from build123d import *

# Parameters (mm, degrees)
F1_DEPTH       = 10
F3_DEPTH       = 10.001
F5_D           = 8.5
F5_CBORE_D     = 11
F5_CBORE_DEPTH = 2
F4_R           = 1.895
F6_DEPTH       = 1.5
F7_R           = 2
F9_DEPTH       = 4


with BuildPart() as f1:
    # F0 (on Front) → F1 (new body, symmetric)
    with BuildSketch(Plane.XZ):
        with BuildLine():
            Line((30, 51.9615242271), (0, 0))
            Line((0, 0), (130, 0))
            Line((130, 0), (130, 10))
            Line((130, 10), (88.031548244, 10))
            ThreePointArc((88.031548244, 10), (82.855167342, 10.6814834742), (78.031548244, 12.6794919243))
            Line((78.031548244, 12.6794919243), (60.9383223748, 22.5482704812))
            Line((60.9383223748, 22.5482704812), (62.1883223748, 24.7133339907))
            Line((62.1883223748, 24.7133339907), (44.8678142991, 34.7133339907))
            Line((44.8678142991, 34.7133339907), (43.6178142991, 32.5482704812))
            Line((43.6178142991, 32.5482704812), (26.2973062234, 42.5482704812))
            Line((26.2973062234, 42.5482704812), (31.2990381057, 51.2115242271))
            Line((31.2990381057, 51.2115242271), (30, 51.9615242271))
        make_face()
        with BuildLine():
            ThreePointArc((78.2347422219, 10.8301270189), (80.5643713533, 5.2059047745), (75.7347422219, 1.5))
            Line((75.7347422219, 1.5), (27.3774332424, 1.5))
            Line((27.3774332424, 1.5), (13.1251234055, 9.7387149337))
            ThreePointArc((13.1251234055, 9.7387149337), (10.7974587698, 12.7747007163), (11.2973058678, 16.5675077516))
            Line((11.2973058678, 16.5675077516), (23.0473062234, 36.9191053566))
            ThreePointArc((23.0473062234, 36.9191053566), (26.0833380169, 39.2487344881), (29.8774332424, 38.7492323755))
            Line((29.8774332424, 38.7492323755), (78.2347422219, 10.8301270189))
        make_face(mode=Mode.SUBTRACT)
    extrude(amount=F1_DEPTH, both=True)

    # F2 (on face) → F3 (cut, through all)
    with BuildSketch(Plane.XY.offset(10)):
        with BuildLine():
            Line((130, -10), (130, -5))
            Line((130, -5), (95, -5))
            ThreePointArc((95, -5), (92.2613872125, -6.7752551286), (92.7639320225, -10))
            Line((92.7639320225, -10), (130, -10))
        make_face()
        with BuildLine():
            ThreePointArc((92.7639320225, 10), (92.2613872125, 6.7752551286), (95, 5))
            Line((95, 5), (130, 5))
            Line((130, 5), (130, 10))
            Line((130, 10), (92.7639320225, 10))
        make_face()
        with BuildLine():
            Line((130, -3), (130, 3))
            Line((130, 3), (113, 3))
            ThreePointArc((113, 3), (110, 0), (113, -3))
            Line((113, -3), (130, -3))
        make_face()
    extrude(amount=-F3_DEPTH, mode=Mode.SUBTRACT)

    # F5 (through all)
    with Locations(Plane(origin=(0, 0, 0), x_dir=(0, -1, 0), z_dir=(-0.8660254038, 0, 0.5))):
        with Locations((0, 7.5)):
            CounterBoreHole(F5_D / 2, F5_CBORE_D / 2, F5_CBORE_DEPTH)

    # F4 (on face) → F6 (cut, through all)
    with BuildSketch(Plane(origin=(0, 0, 0), x_dir=(0, -1, 0), z_dir=(-0.8660254038, 0, 0.5))):
        with Locations((-5, 39)):
            Circle(F4_R)
        with Locations((5, 39)):
            Circle(F4_R)
        with Locations((-5, 32)):
            Circle(F4_R)
        with Locations((5, 32)):
            Circle(F4_R)
        with Locations((-5, 25)):
            Circle(F4_R)
        with Locations((5, 25)):
            Circle(F4_R)
    extrude(amount=-F6_DEPTH, mode=Mode.SUBTRACT)

    # F7
    f7_edges = [f1.edges().sort_by_distance(p)[0] for p in [
        (43.617814, 0, 32.54827),
        (60.938322, 0, 22.54827),
        (26.297306, 0, 42.54827),
    ]]
    fillet(f7_edges, radius=F7_R)

    # F8 (on face) → F9 (cut, through all)
    with BuildSketch(Plane(origin=(26.2482681178, 0, 45.4633339907), x_dir=(0.8660254038, 0, -0.5), z_dir=(0.5, 0, 0.8660254038))):
        with BuildLine():
            ThreePointArc((28, 4), (24, 0), (28, -4))
            Line((28, -4), (35, -4))
            ThreePointArc((35, -4), (39, 0), (35, 4))
            Line((35, 4), (28, 4))
        make_face()
    extrude(amount=-F9_DEPTH, mode=Mode.SUBTRACT)


solid = f1.part
Part model, mm, in its own coordinate system. A direction names the side the tool comes from. Round coordinates to 2 decimals unless told otherwise and drop trailing zeros. Loops run counter-clockwise (first coordinate to the right, second up) from the corner with the lowest first, then second, coordinate; pieces in that order, holes last. Notation, with made-up numbers: (-8.5, 72.5) - (27.5, 72.5) arc R23 ccw to (27.5, 80.5) - close; hole circle Ø8 at (-8.75, -4.5). An arc over 180 degrees is marked (long way). Answer as a JSON object with one key per item and string values.
Item 1: Tool access for faces 5 (the face through (113, -5, 5)), 6 (the face through (26.03, -0.14, 39.234)), 7 (the face through (61.733, -0.14, 22.784)), 8 (the face through (59.04, -0.09, 24.26)), 9 (the face through (122, 3, 5)): list every direction of +Z, -Z, +X, -X, +Y, -Y with a clear straight run to the whole face (end or side of a thin tool).
Output:
{"face 5": "+Z, -Z, +X, -Y", "face 6": "+Y, -Y", "face 7": "+X, +Y, -Y", "face 8": "+Z", "face 9": "+Z, -Z, +X"}
Item 2: Band-saw the part on D-D on x = 108.5. List the corners of the cut face in (y, z).
Output:
{"outline": "(-5, 0) - (5, 0) - (5, 10) - (-5, 10) - close"}
Item 3: Band-saw the part on A-A on x = 66. List the corners of the cut face in (y, z), plus the area to 3 significant figures.
Output:
{"outline": "(-10, 0) - (10, 0) - (10, 1.5) - (-10, 1.5) - close; (-10, 17.89) - (10, 17.89) - (10, 19.63) - (-10, 19.63) - close", "area": "64.6 mm2"}
Item 4: Band-saw the part on C-C on y = 8.5. List the corners of the cut face in (x, z), plus the area to 3 significant figures.
Output:
{"outline": "(0, 0) - (92.04, 0) - (92.04, 10) - (88.03, 10) arc R20 cw to (78.03, 12.68) - (62.67, 21.55) arc R2 cw to (61.94, 24.28) - (62.19, 24.71) - (44.87, 34.71) - (44.62, 34.28) arc R2 cw to (41.89, 33.55) - (28.03, 41.55) arc R2 cw to (27.3, 44.28) - (31.3, 51.21) - (30, 51.96) - close; hole (11.3, 16.57) arc R5 ccw to (13.13, 9.74) - (27.38, 1.5) - (75.73, 1.5) arc R5 ccw to (78.23, 10.83) - (29.88, 38.75) arc R5 ccw to (23.05, 36.92) - close", "area": "622 mm2"}
Item 5: Pin check, flat tips, straight feed: pin 1 (1 mm diameter, centred on y = 2, z = 32.5, fed in from +X); pin 2 (8 mm diameter, centred on y = 3.5, z = 11.5, fed in from -X); pin 3 (5 mm diameter, centred on x = 118.5, z = 5, fed in from -Y). Stop position of each tip, or through.
Output:
{"pin 1": "x = 47.57", "pin 2": "x = 4.56", "pin 3": "y = -5"}
Item 6: Pull direction X, two halves, no side cores. Call faces 1 (the face through (46.05, 0.09, 31.76)), 2 (the face through (43, -10, 1)), 3 (the face through (43.382, 0.14, 33.343)), 4 (the face through (52, 0, 1.5)): pulls with the +X half, pulls with the -X half, needs draft (parallel to the pull), parting line crosses it, or undercut.
Output:
{"face 1": "pulls with the +X half", "face 2": "needs draft", "face 3": "undercut", "face 4": "undercut"}
Item 7: Wall check: L1, parallel to Z at x = 28, y = -6; L2, parallel to Z at x = 27.5, y = -1.25; L3, parallel to Z at x = 97, y = -2.75. Give the ranges that are in metal, low to high.
Output:
{"L1": "0 to 1.5, 39.38 to 41.57, 45.5 to 48.5", "L2": "0 to 1.5, 39.42 to 41.99, 44.63 to 47.63", "L3": "0 to 10"}
